from build123d import *

# Parameters (mm, degrees)
SKETCH1_W           = 132
SKETCH1_H           = 85.5
BOSS_EXTRUDE1_DEPTH = 5
BOSS_EXTRUDE3_DEPTH = 5
FILLET1_R           = 2
SKETCH5_R           = 2
CUT_EXTRUDE1_DEPTH  = 7
SKETCH6_R           = 3.75
CUT_EXTRUDE2_DEPTH  = 2
FILLET2_R           = 7
SKETCH7_W           = 101.652764849
SKETCH7_H           = 21.79377459
CUT_EXTRUDE3_DEPTH  = 90
CUT_EXTRUDE4_DEPTH  = 5
BOSS_EXTRUDE4_DEPTH = 2.2
CUT_EXTRUDE5_DEPTH  = 1.1


with BuildPart() as part:
    # Sketch1 → Boss-Extrude1 (new body)
    with BuildSketch(Plane(origin=(0, 0, 0), x_dir=(1, 0, 0), z_dir=(0, 1, 0))):
        Rectangle(SKETCH1_W, SKETCH1_H)
    extrude(amount=BOSS_EXTRUDE1_DEPTH)

    # Sketch4 → Boss-Extrude3 (add)
    with BuildSketch(Plane(origin=(0, 5, 0), x_dir=(1, 0, 0), z_dir=(0, 1, 0))):
        with BuildLine():
            Line((-66, 15.5), (-66, 8))
            ThreePointArc((-66, 8), (-69.75, 11.75), (-66, 15.5))
        make_face()
        with BuildLine():
            Line((-66, -23.5), (-66, -31))
            ThreePointArc((-66, -31), (-69.75, -27.25), (-66, -23.5))
        make_face()
        with BuildLine():
            Line((66, -31), (66, -23.5))
            ThreePointArc((66, -23.5), (69.75, -27.25), (66, -31))
        make_face()
        with BuildLine():
            Line((66, 8), (66, 15.5))
            ThreePointArc((66, 15.5), (69.75, 11.75), (66, 8))
        make_face()
    extrude(amount=-BOSS_EXTRUDE3_DEPTH)

    # Fillet1
    fillet1_edges = [part.edges().sort_by_distance(p)[0] for p in [
        (-66, 2.5, -8),
        (-66, 2.5, -15.5),
        (-66, 2.5, 31),
        (-66, 2.5, 23.5),
        (66, 2.5, 23.5),
        (66, 2.5, 31),
        (66, 2.5, -15.5),
        (66, 2.5, -8),
    ]]
    fillet(fillet1_edges, radius=FILLET1_R)

    # Sketch5 → Cut-Extrude1 (cut)
    with BuildSketch(Plane(origin=(0, 5, 0), x_dir=(1, 0, 0), z_dir=(0, 1, 0))):
        with Locations(Location((-66, 11.75, 0), (0, 0, 270))):
            Circle(SKETCH5_R)
        with Locations(Location((66, 11.75, 0), (0, 0, 270))):
            Circle(SKETCH5_R)
        with Locations(Location((66, -27.25, 0), (0, 0, 270))):
            Circle(SKETCH5_R)
        with Locations(Location((-66, -27.25, 0), (0, 0, 270))):
            Circle(SKETCH5_R)
    extrude(amount=-CUT_EXTRUDE1_DEPTH, mode=Mode.SUBTRACT)

    # Sketch6 → Cut-Extrude2 (cut)
    with BuildSketch(Plane(origin=(0, 5, 0), x_dir=(1, 0, 0), z_dir=(0, 1, 0))):
        with Locations((-66, 11.75)):
            Circle(SKETCH6_R)
        with Locations((-66, -27.25)):
            Circle(SKETCH6_R)
        with Locations((66, -27.25)):
            Circle(SKETCH6_R)
        with Locations((66, 11.75)):
            Circle(SKETCH6_R)
    extrude(amount=-CUT_EXTRUDE2_DEPTH, mode=Mode.SUBTRACT)

    # Fillet2
    fillet2_edges = [part.edges().sort_by_distance(p)[0] for p in [
        (-66, 2.5, -42.75),
        (66, 2.5, -42.75),
    ]]
    fillet(fillet2_edges, radius=FILLET2_R)

    # Sketch7 → Cut-Extrude3 (cut)
    with BuildSketch(Plane.XY.offset(42.75)):
        with Locations((26.626382425, 4.310675182)):
            Rectangle(SKETCH7_W, SKETCH7_H)
    extrude(amount=-CUT_EXTRUDE3_DEPTH, mode=Mode.SUBTRACT)

    # Mirror1: part across plane


with BuildPart() as part_1:
    add(part.part)
    add(part.part.mirror(Plane(origin=(-24.2, 15.207562477, -47.25), x_dir=(0, 0, 1), z_dir=(-1, 0, 0))))

    # Sketch9 → Cut-Extrude4 (cut)
    with BuildSketch(Plane(origin=(0, 5, 0), x_dir=(1, 0, 0), z_dir=(0, 1, 0))):
        Polygon((-44.8, -26.35), (-44.8, 38.35), (-61.8, 38.35), (-61.8, -26.35), (-61.8, -35.65), (-44.8, -35.65), align=None)
        Polygon((-34.8, -25.15), (-23.1, -25.15), (-13.8, -25.15), (-13.8, -8.65), (-13.8, 9.35), (-23.1, 9.35), (-34.8, 9.35), (-34.8, -8.65), align=None)
        Polygon((13.2, -26.35), (13.2, -35.65), (-3.8, -35.65), (-3.8, -26.35), (-3.8, 25.35), (13.2, 25.35), align=None)
        Polygon((-22.6, 29.85), (-42.5, 29.85), (-42.5, 20.05), (-6.1, 20.05), (-6.1, 29.85), align=None)
    extrude(amount=-CUT_EXTRUDE4_DEPTH, mode=Mode.SUBTRACT)

    # Sketch11 → Boss-Extrude4 (add)
    with BuildSketch(Plane.XZ):
        Polygon((14.1, 42.75), (-62.7, 42.75), (-62.7, -32.810601847), (-61.8, -32.810601847), (-61.8, 40.250110422), (13.2, 40.250110422), (13.2, -32.810601847), (14.1, -32.810601847), align=None)
    extrude(amount=BOSS_EXTRUDE4_DEPTH)

    # Sketch12 → Cut-Extrude5 (cut)
    with BuildSketch(Plane.XY.offset(42.75)):
        Polygon((-66, 0), (-62.7, 0), (-62.7, -2.2), (14.1, -2.2), (14.1, 0), (17.6, 0), (17.6, 5), (-66, 5), align=None)
    extrude(amount=-CUT_EXTRUDE5_DEPTH, mode=Mode.SUBTRACT)


solid = part_1.part
Can you work these out from the model? Positions are in its coordinate system, mm. A direction names the side the tool comes from. Give positions to 0.01 mm unless a question says otherwise; leave off trailing zeros. Order: outer loops, then holes, each group sorted by start corner. A loop starts at its lowest first (then second) coordinate and runs counter-clockwise, first axis right, second up. Notation, with made-up numbers: M 55,8 L 81,8 A24 cw 81,43 Z; hole C 32.5,35 d4. An arc over 180 degrees is marked long. Use one line per item in the form item = value.
Item 1: If we section it at B-B, the plane z = -11.75: Write out the boundary of the cut face in (x, y), and give its area (3 significant figures).
Values follow:
outline = M -69.75,0 L -68,0 L -68,3 L -69.75,3 Z; M -64,0 L -62.7,0 L -62.7,-2.2 L -61.8,-2.2 L -61.8,5 L -62.25,5 L -62.25,3 L -64,3 Z; M -44.8,0 L -3.8,0 L -3.8,5 L -44.8,5 Z; M 13.2,-2.2 L 14.1,-2.2 L 14.1,0 L 15.6,0 L 15.6,3 L 13.85,3 L 13.85,5 L 13.2,5 Z; M 19.6,0 L 21.35,0 L 21.35,3 L 19.6,3 Z
area = 235 mm^2
Item 2: If we section it at D-D, the plane z = -3: Write out the boundary of the cut face in (x, y), and give its area (3 significant figures).
Values follow:
outline = M -66,0 L -62.7,0 L -62.7,-2.2 L -61.8,-2.2 L -61.8,5 L -66,5 Z; M -44.8,0 L -34.8,0 L -34.8,5 L -44.8,5 Z; M -13.8,0 L -3.8,0 L -3.8,5 L -13.8,5 Z; M 13.2,-2.2 L 14.1,-2.2 L 14.1,0 L 17.6,0 L 17.6,5 L 13.2,5 Z
area = 147 mm^2
Item 3: If we section it at A-A, the plane x = 2.5: Write out the boundary of the cut face in (y, z).
Values follow:
outline = M -2.2,40.25 L 0,40.25 L 0,35.65 L 5,35.65 L 5,41.65 L -2.2,41.65 Z; M 0,-42.75 L 5,-42.75 L 5,-25.35 L 0,-25.35 Z
Item 4: If I drill on line 1 along X through (y, z) = (1.8, -11.75); line 2 along X through (y, z) = (3.7, -11.75); line 3 along X through (y, z) = (2, 15.5), over which ranges is the centre line in solid material (lowest first)? Write a range as [from, to].
Values follow:
line_1 = [-69.75, -68], [-64, -61.8], [-44.8, -3.8], [13.2, 15.6], [19.6, 21.35]
line_2 = [-62.25, -61.8], [-44.8, -3.8], [13.2, 13.85]
line_3 = [-66, -61.8], [-44.8, -34.8], [-13.8, -3.8], [13.2, 17.6]
Item 5: Will these pins go through, and if not, where does the flat tip stop? pin 1 Ø1 at (y, z) = (3.5, -18) entering from -X; pin 2 Ø1.5 at (y, z) = (1.5, 7.5) entering from +X; pin 3 Ø2 at (x, z) = (-6, -22) entering from -Y; pin 4 Ø8 at (x, z) = (-67, 26) entering from +Y.
Values follow:
pin_1 = -66
pin_2 = 17.6
pin_3 = 0
pin_4 = 5
Item 6: Thinking about a two-plate mould opening in X: for faces 4 (the flat face through (17.6, 2, 37)), 5 (the cylindrical face through (-66.37, 2.46, 23.02)), 6 (the flat face through (-24, 3, 25.15)), which applies, pulls with the +X half, pulls with the -X half, needs draft (parallel to the pull), parting line crosses it, or undercut?
Values follow:
face_4 = pulls with the +X half
face_5 = pulls with the -X half
face_6 = undercut
Item 7: If we section it at C-C, the plane x = -15.5: Write out the boundary of the cut face in (y, z), and give its area (3 significant figures).
Values follow:
outline = M -2.2,40.25 L 0,40.25 L 0,25.15 L 5,25.15 L 5,41.65 L -2.2,41.65 Z; M 0,-42.75 L 5,-42.75 L 5,-29.85 L 0,-29.85 Z; M 0,-20.05 L 5,-20.05 L 5,-9.35 L 0,-9.35 Z
area = 204 mm^2
Item 8: For faces 1 (the cylindrical face through (-64, 2.54, -40.65)), 2 (the flat face through (-66, 2, 37)), 3 (the flat face through (-53, 3, -38.35)), which set-ups out of +Z, -Z, +X, -X, +Y, -Y let a thin tool reach every point of the face, with its end or its side?
Values follow:
face_1 = -Z, -X, +Y, -Y
face_2 = +Z, -X, +Y, -Y
face_3 = +Y, -Y
